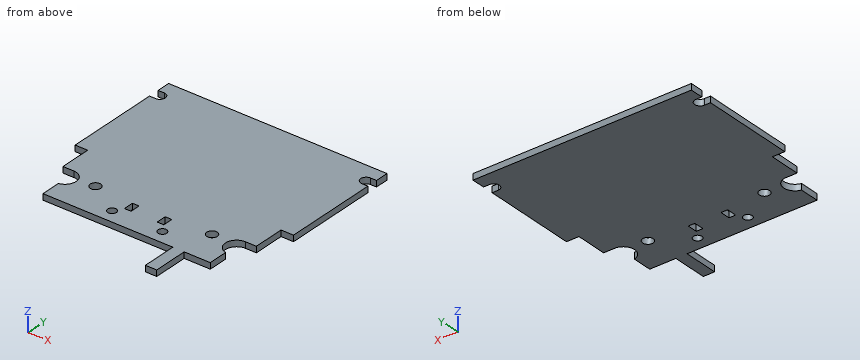
from build123d import *

# Parameters (mm, degrees)
SKIZZE1_R                       = 1.35
SKIZZE1_R_2                     = 1.1
SKIZZE1_W                       = 1.7
SKIZZE1_H                       = 2.6
AUFSATZ_LINEAR_AUSTRAGEN1_DEPTH = 1.55


with BuildPart() as part:
    # Skizze1 → Aufsatz-Linear austragen1 (new body)
    with BuildSketch(Plane.XY):
        with BuildLine():
            Line((-28, 23.303403096), (-28, 26.703403096))
            Line((-28, 26.703403096), (28, 26.703403096))
            Line((28, 26.703403096), (28, 23.303403096))
            Line((28, 23.303403096), (26.4, 23.303403096))
            ThreePointArc((26.4, 23.303403096), (25.05, 21.903403096), (26.4, 20.503403096))
            Line((26.4, 20.503403096), (28, 20.503403096))
            Line((28, 20.503403096), (28, -3.596596904))
            Line((28, -3.596596904), (24.8, -3.596596904))
            Line((24.8, -3.596596904), (24.8, -11.596596904))
            Line((24.8, -11.596596904), (22, -11.596596904))
            ThreePointArc((22, -11.596596904), (19.136763195, -14.196854756), (21.45, -17.296596904))
            Line((21.45, -17.296596904), (21.45, -22.296596904))
            Line((21.45, -22.296596904), (14.75, -22.296596904))
            Line((14.75, -22.296596904), (14.75, -31.196596904))
            Line((14.75, -31.196596904), (11.85, -31.196596904))
            Line((11.85, -31.196596904), (11.85, -22.296596904))
            Line((11.85, -22.296596904), (-21.45, -22.296596904))
            Line((-21.45, -22.296596904), (-21.45, -17.296596904))
            ThreePointArc((-21.45, -17.296596904), (-19.136763195, -14.196854756), (-22, -11.596596904))
            Line((-22, -11.596596904), (-24.8, -11.596596904))
            Line((-24.8, -11.596596904), (-24.8, -3.596596904))
            Line((-24.8, -3.596596904), (-28, -3.596596904))
            Line((-28, -3.596596904), (-28, 20.503403096))
            Line((-28, 20.503403096), (-26.4, 20.503403096))
            ThreePointArc((-26.4, 20.503403096), (-25.05, 21.903403096), (-26.4, 23.303403096))
            Line((-26.4, 23.303403096), (-28, 23.303403096))
        make_face()
        with Locations((14.95, -13.496596904)):
            Circle(SKIZZE1_R, mode=Mode.SUBTRACT)
        with Locations((-14.95, -13.496596904)):
            Circle(SKIZZE1_R, mode=Mode.SUBTRACT)
        with Locations((6.45, -18.852047487)):
            Circle(SKIZZE1_R_2, mode=Mode.SUBTRACT)
        with Locations((-6.45, -18.852047487)):
            Circle(SKIZZE1_R_2, mode=Mode.SUBTRACT)
        with Locations((-4.2, -15.345681582)):
            Rectangle(SKIZZE1_W, SKIZZE1_H, mode=Mode.SUBTRACT)
        with Locations((4.2, -15.345681582)):
            Rectangle(SKIZZE1_W, SKIZZE1_H, mode=Mode.SUBTRACT)
    extrude(amount=AUFSATZ_LINEAR_AUSTRAGEN1_DEPTH)


solid = part.part
The listing builds one solid part. Answer for the finished solid, in the listing's coordinates (mm). Give positions to 0.01 mm unless a question says otherwise; leave off trailing zeros. Loops run counter-clockwise (first coordinate to the right, second up) from the corner with the lowest first, then second, coordinate; pieces in that order, holes last. Notation, with made-up numbers: M -22,5.5 L 15,5.5 A18 ccw 15,16.5 Z; hole C -2.75,75 d10. An arc over 180 degrees is marked long. Answer as CSV lines item,"result".
Item 1: Straight lines are drawn through the part: line 1 along Y through (x, z) = (-6.45, 0.6); line 2 along Y through (x, z) = (-14.95, 0.7); line 3 along X through (y, z) = (-27.5, 1.15). For each, find the intervals that lie inside material, in ascending order. Write a range as [from, to].
Values follow:
line 1,"y = [-22.3, -19.95], [-17.75, 26.7]"
line 2,"y = [-22.3, -14.85], [-12.15, 26.7]"
line 3,"x = [11.85, 14.75]"
Item 2: The part is cut by section B-B (y = -6.5). Give the vertices of the cut face in (x, z), and give its area (3 significant figures).
Values follow:
outline,"M -24.8,0 L 24.8,0 L 24.8,1.55 L -24.8,1.55 Z"
area,"76.9 mm^2"
Item 3: The part is cut by section C-C (x = -4). Give the vertices of the cut face in (y, z).
Values follow:
outline,"M -22.3,0 L -16.65,0 L -16.65,1.55 L -22.3,1.55 Z; M -14.05,0 L 26.7,0 L 26.7,1.55 L -14.05,1.55 Z"
Item 4: Given pin 1 Ø0.5 at (y, z) = (-16, 0.5) entering from +X; pin 2 Ø0.5 at (y, z) = (-15.5, 1) entering from -X; pin 3 Ø0.5 at (y, z) = (-24.5, 1) entering from +X, each flat-ended and moving along its own axis, determine where each tip first touches the part or whether it passes through.
Values follow:
pin 1,"stops at x = 19.74"
pin 2,"stops at x = -19.42"
pin 3,"stops at x = 14.75"
Item 5: The part is cut by section D-D (z = 0.45). Give the number of separate pieces and of enclosed holes in the cut face, and give its area (3 significant figures).
Values follow:
separate pieces,"1"
enclosed holes,"6"
area,"2,520 mm^2"
Item 6: The part is cut by section A-A (x = -14.95). Give the vertices of the cut face in (y, z).
Values follow:
outline,"M -22.3,0 L -14.85,0 L -14.85,1.55 L -22.3,1.55 Z; M -12.15,0 L 26.7,0 L 26.7,1.55 L -12.15,1.55 Z"
